Input: part model. Units: mm. Frame: model coordinates. Face numbers are marked on the shaded views. Round coordinates to 2 decimals unless told otherwise and drop trailing zeros. Loops run counter-clockwise (first coordinate to the right, second up) from the corner with the lowest first, then second, coordinate; pieces in that order, holes last.
1) Section A-A, the plane y = 10. Return loops of the section in (x, z).
2) First-contact query: pin 1 (1.5 mm diameter, centred on y = 20, z = -4.5, fed in from +X); pin 2 (0.6 mm diameter, centred on x = 5, z = -1, fed in from +Y); pin 3 (2 mm diameter, centred on x = 4, y = 12, fed in from -Z). Flat tips, straight axial feed; report the tip coordinate or a pass-through.
3) Ray query, line 1 along Z through (x, y) = (0, 10.75); line 2 along X through (y, z) = (28.5, -4). Return the intervals inside material, ascending.
4) Draft query along X for the marked faces 1, 2, 3 and 4. Return one class per face: pulls with the +X half, pulls with the -X half, needs draft (parallel to the pull), parting line crosses it, or undercut.
5) Section B-B, the plane y = 26.5. Return loops of the section in (x, z).
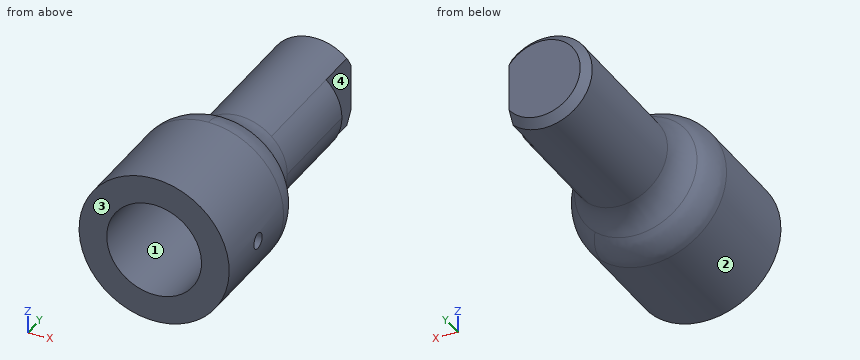
from build123d import *

# Parameters (mm, degrees)
SKETCH1_R               = 9.5
SKETCH1_R_2             = 6
BOSS_EXTRUDE1_DEPTH     = 16
BOSS_EXTRUDE2_START     = 14
BOSS_EXTRUDE2_DEPTH     = 26
BOSS_EXTRUDE5_START     = 14
BOSS_EXTRUDE5_DEPTH     = 20
CUT_EXTRUDE1_REACH      = 44.196
CUT_EXTRUDE1_END_RADIUS = 9.5
SKETCH2_R               = 1
CHAMFER1_SIZE           = 1
FILLET2_R               = 5
FILLET3_R               = 5


with BuildPart() as part:
    # Sketch1 → Boss-Extrude1 (new body)
    with BuildSketch(Plane(origin=(0, 0, 0), x_dir=(1, 0, 0), z_dir=(0, 1, 0))):
        with Locations(Location((0, 0, 0), (0, 0, 270))):
            Circle(SKETCH1_R)
        with Locations(Location((0, 0, 0), (0, 0, 270))):
            Circle(SKETCH1_R_2, mode=Mode.SUBTRACT)
    extrude(amount=BOSS_EXTRUDE1_DEPTH)



with BuildPart() as body_2:
    # Sketch1<3> → Boss-Extrude2 (new body)
    with BuildSketch(Plane(origin=(0, 0, 0), x_dir=(1, 0, 0), z_dir=(0, 1, 0)).offset(BOSS_EXTRUDE2_START)):
        with BuildLine():
            Line((4, -4.472135955), (4, 4.472135955))
            ThreePointArc((4, 4.472135955), (-6, 0), (4, -4.472135955))
        make_face()
    extrude(amount=BOSS_EXTRUDE2_DEPTH)


with BuildPart() as part_1:
    add(part.part)

    add(body_2.part)  # Boss-Extrude5 merges body 2
    # Sketch1<5> → Boss-Extrude5 (add)
    with BuildSketch(Plane(origin=(0, 0, 0), x_dir=(1, 0, 0), z_dir=(0, 1, 0)).offset(BOSS_EXTRUDE5_START)):
        with BuildLine():
            ThreePointArc((6, 0), (5.477225575, 2.449489743), (4, 4.472135955))
            Line((4, 4.472135955), (4, -4.472135955))
            ThreePointArc((4, -4.472135955), (5.477225575, -2.449489743), (6, 0))
        make_face()
        with BuildLine():
            Line((4, -4.472135955), (4, 4.472135955))
            ThreePointArc((4, 4.472135955), (-6, 0), (4, -4.472135955))
        make_face()
    extrude(amount=BOSS_EXTRUDE5_DEPTH)

    # Cut-Extrude1: up to this cylinder (the profile starts inside it)
    cut_extrude1_end = Plane(origin=(0, 7, 0), z_dir=(0, -1, 0)) * Cylinder(CUT_EXTRUDE1_END_RADIUS, 108.392, mode=Mode.PRIVATE)
    # Sketch2 → Cut-Extrude1 (cut, up to the surface)
    with BuildSketch(Plane(origin=(0, 0, 0), x_dir=(0, 0, -1), z_dir=(1, 0, 0)), mode=Mode.PRIVATE) as cut_extrude1_sk1:
        with Locations(Location((0, 7, 0), (0, 0, 180))):
            Circle(SKETCH2_R)
    cut_extrude1_tool1 = extrude(cut_extrude1_sk1.sketch, amount=CUT_EXTRUDE1_REACH, mode=Mode.PRIVATE) & cut_extrude1_end
    add(cut_extrude1_tool1.solids().sort_by_distance((0, 7, 0))[0], mode=Mode.SUBTRACT)

    # Chamfer1
    chamfer1_edges = [part_1.edges().sort_by_distance(p)[0] for p in [
        (-6, 40, 0),
    ]]
    chamfer(chamfer1_edges, length=CHAMFER1_SIZE)

    # Fillet2
    # the kernel refuses this fillet: 5 mm, written as the material it adds along each edge
    with BuildSketch(Plane(origin=(0, 16, 0), x_dir=(0.6666666666667012, 0, -0.745355992499899), z_dir=(-0.745355992499899, 0, -0.6666666666667012))) as fillet2_piece_1:
        with BuildLine():
            CenterArc((11, -4.769696007), FILLET2_R, 107.457603124, 72.542396876)
            Line((9.5, 0), (9.47, 0.09539392))
            ThreePointArc((9.47, 0.09539392), (7.75, 0.1), (6, 0.1))
            Line((6, 0.1), (5.9, 0))
            Line((5.9, 0), (5.9, -4.769696007))
            Line((5.9, -4.769696007), (6, -4.769696007))
        make_face()
    revolve(axis=Axis((0, 16, 0), (0, -1, 0)))

    # Fillet3
    fillet3_edges = [part_1.edges().sort_by_distance(p)[0] for p in [
        (8.87463741, 16, 3.389809853),
    ]]
    fillet(fillet3_edges, radius=FILLET3_R)


solid = part_1.part
Final values:
1. outline: circle Ø19 at (0, 0); hole circle Ø12 at (0, 0)
2. pin 1: stops at x = 4.78
2. pin 2: stops at y = 34
2. pin 3: stops at z = -9.01
3. line 1: z = -9.5 to -6, 6 to 9.5
3. line 2: x = -4.47 to 4.47
4. face 1: undercut
4. face 2: parting line crosses it
4. face 3: needs draft
4. face 4: pulls with the +X half
5. outline: circle Ø12 at (0, 0)
